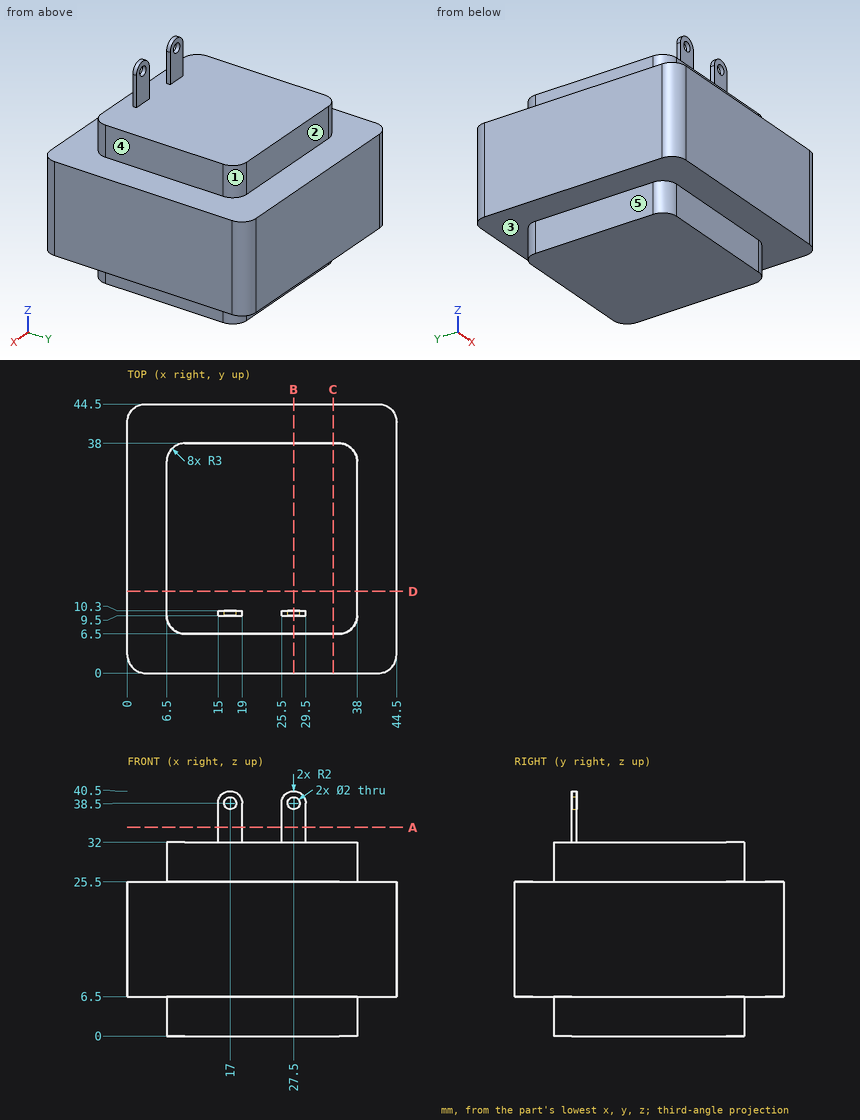
Study the drawing (mm; zero at the part's minimum x, y, z) and answer. A direction names the side the tool comes from. Coordinates: 2 decimals unless noted, no trailing zeros. Order: outer loops, then holes, each group sorted by start corner. A loop starts at its lowest first (then second) coordinate and runs counter-clockwise, first axis right, second up. Notation, with made-up numbers: (-31.5, 82) -> (-25.5, 82) arc R25 cw to (-25.5, 112) -> close; hole circle Ø5 at (-36.5, -14). An arc over 180 degrees is marked (long way). Answer in a Markdown table with one row per item. Add a question column.
Item 1: Find the intervals of material crossed by L1, parallel to X at y = 10.05, z = 38.5; L2, parallel to X at y = 10, z = 38; L3, parallel to Z at x = 10, y = 32.5, in increasing order. Write a range as from..to.
Item 2: Which of the six approach directions +Z, -Z, +X, -X, +Y, -Y give full straight-line access (tool end or side, diameter ignored) to the marked faces 1, 2, 3, 4 and 5?
Item 3: Find section C-C (x = 34). Write down the section's boundary in (y, z), then the cut area to 4 significant figures.
Item 4: Find section B-B (x = 27.5). Write down the section's boundary in (y, z).
Item 5: Each of these flat-tipped pins is pushed along its axis until it touches: P1, Ø0.6, axis at y = 10, z = 33.5, coming from the -X side; P2, Ø2, axis at x = 27, z = 36, coming from the +Y side; P3, Ø3, axis at x = 19.5, z = 2, coming from the -Y side. Where does it stop, or does it pass through?
Item 6: Find section A-A (z = 34.5). Write down the section's boundary in (x, y).
Result set:
| question | item | result |
|---|---|---|
| 1 | L1 | x = 15..16, 18..19, 25.5..26.5, 28.5..29.5 |
| 1 | L2 | x = 15..16.13, 17.87..19, 25.5..26.63, 28.37..29.5 |
| 1 | L3 | z = 0..32 |
| 2 | face 1 | +Z, +X, +Y |
| 2 | face 2 | +Z, +X, -X, +Y |
| 2 | face 3 | -Z |
| 2 | face 4 | +Z, +X, +Y, -Y |
| 2 | face 5 | -Z, -X, +Y, -Y |
| 3 | outline | (0, 6.5) -> (6.5, 6.5) -> (6.5, 0) -> (38, 0) -> (38, 6.5) -> (44.5, 6.5) -> (44.5, 25.5) -> (38, 25.5) -> (38, 32) -> (6.5, 32) -> (6.5, 25.5) -> (0, 25.5) -> close |
| 3 | area | 1,255 mm² |
| 4 | outline | (0, 6.5) -> (6.5, 6.5) -> (6.5, 0) -> (38, 0) -> (38, 6.5) -> (44.5, 6.5) -> (44.5, 25.5) -> (38, 25.5) -> (38, 32) -> (10.3, 32) -> (10.3, 37.5) -> (9.5, 37.5) -> (9.5, 32) -> (6.5, 32) -> (6.5, 25.5) -> (0, 25.5) -> close; (9.5, 39.5) -> (10.3, 39.5) -> (10.3, 40.5) -> (9.5, 40.5) -> close |
| 5 | P1 | stops at x = 15 |
| 5 | P2 | stops at y = 10.3 |
| 5 | P3 | stops at y = 6.5 |
| 6 | outline | (15, 9.5) -> (19, 9.5) -> (19, 10.3) -> (15, 10.3) -> close; (25.5, 9.5) -> (29.5, 9.5) -> (29.5, 10.3) -> (25.5, 10.3) -> close |
